Check sheet for the modelled part. Datum: model origin and axes. Units: mm. Face numbers are marked on the shaded views. Round coordinates to 2 decimals unless told otherwise and drop trailing zeros. Loops run counter-clockwise (first coordinate to the right, second up) from the corner with the lowest first, then second, coordinate; pieces in that order, holes last. Notation, with made-up numbers: (28, 49.25) -> (53, 49.25) arc R32 cw to (53, 75.25) -> close; hole circle Ø2 at (64, 20.25). An arc over 180 degrees is marked (long way). One line per item, written item: value. Start each with the question number.
1. Cross-section at C-C on y = 0.6. Record the cut outline in (x, z) (3 decimals), then the cut area to 3 significant figures.
2. Material ranges on L1, parallel to Z at x = 52, y = 1.9 (3 decimals); L2, parallel to X at y = 1.85, z = -8.25; L3, parallel to Z at x = 51.5, y = 0.65, recorded low to high.
3. Release check for a two-part mould opening along Z. For the marked faces 1 and 2 record: +Z half, -Z half, draft (parallel to the pull), parting line (faces both ways), or undercut.
4. Cross-section at A-A on x = 8. Record the cut outline in (y, z) (3 decimals), then the cut area to 3 significant figures.
5. Cross-section at B-B on z = -11. Record the cut outline in (x, y), then the cut area to 3 significant figures.
6. Cross-section at D-D on x = 51.5. Record the cut outline in (y, z).
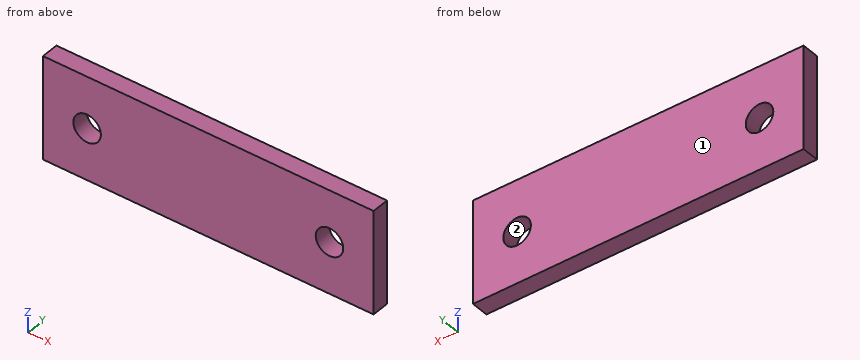
from build123d import *

# Parameters (mm, degrees)
SKETCH1_W                 = 60
SKETCH1_H                 = 18.67
BOSS_EXTRUDE1_DEPTH       = 3.15
F_5_0MM_DOWEL_HOLE1_D     = 5
F_5_0MM_DOWEL_HOLE1_DEPTH = 3.15


with BuildPart() as part:
    # Sketch1 → Boss-Extrude1 (new body)
    with BuildSketch(Plane(origin=(0, 0, 0), x_dir=(1, 0, 0), z_dir=(0, 1, 0))):
        with Locations((30, 9.335)):
            Rectangle(SKETCH1_W, SKETCH1_H)
    extrude(amount=BOSS_EXTRUDE1_DEPTH)

    # Ø5.0mm Dowel Hole1
    with Locations(Plane(origin=(0, 3.15, 0), x_dir=(1, 0, 0), z_dir=(0, 1, 0))):
        with Locations((8, 9.335), (52, 9.335)):
            Hole(F_5_0MM_DOWEL_HOLE1_D / 2, depth=F_5_0MM_DOWEL_HOLE1_DEPTH)


solid = part.part
Taken from the geometry:
1. outline: (0, -18.67) -> (60, -18.67) -> (60, 0) -> (0, 0) -> close; hole circle Ø5 at (8, -9.335); hole circle Ø5 at (52, -9.335)
1. area: 1,080 mm2
2. L1: z = -18.67 to -11.835, -6.835 to 0
2. L2: x = 0 to 5.75, 10.25 to 49.75, 54.25 to 60
2. L3: z = -18.67 to -11.78, -6.89 to 0
3. face 1: draft
3. face 2: undercut
4. outline: (0, -18.67) -> (3.15, -18.67) -> (3.15, -11.835) -> (0, -11.835) -> close; (0, -6.835) -> (3.15, -6.835) -> (3.15, 0) -> (0, 0) -> close
4. area: 43.1 mm2
5. outline: (0, 0) -> (6.14, 0) -> (6.14, 3.15) -> (0, 3.15) -> close; (9.86, 0) -> (50.14, 0) -> (50.14, 3.15) -> (9.86, 3.15) -> close; (53.86, 0) -> (60, 0) -> (60, 3.15) -> (53.86, 3.15) -> close
5. area: 166 mm2
6. outline: (0, -18.67) -> (3.15, -18.67) -> (3.15, -11.78) -> (0, -11.78) -> close; (0, -6.89) -> (3.15, -6.89) -> (3.15, 0) -> (0, 0) -> close
